```python
from build123d import *

# Parameters (mm, degrees)
F0_W     = 7
F0_H     = 5
F0_H_2   = 1
F0_W_2   = 10
F0_W_3   = 5
F0_H_3   = 2.5
F1_DEPTH = 30


with BuildPart() as f1:
    # F0 (on Top) → F1 (new body)
    with BuildSketch(Plane.XY):
        with BuildLine():
            Line((20, 12.5), (20, 17.5))
            Line((20, 17.5), (-13, 17.5))
            Line((-13, 17.5), (-13, 12.5))
            Line((-13, 12.5), (-8.2915619759, 12.5))
            ThreePointArc((-8.2915619759, 12.5), (0, 15), (8.2915619759, 12.5))
            Line((8.2915619759, 12.5), (20, 12.5))
        make_face()
        with Locations((23.5, 15)):
            Rectangle(F0_W, F0_H)
        with Locations((-16.5, 15)):
            Rectangle(F0_W, F0_H)
        with Locations((23.5, 12)):
            Rectangle(F0_W, F0_H_2)
        with BuildLine():
            Line((20, 11.5), (20, 12.5))
            Line((20, 12.5), (8.2915619759, 12.5))
            ThreePointArc((8.2915619759, 12.5), (13.2169101843, 7.0931858273), (15, 0))
            ThreePointArc((15, 0), (13.2169101843, -7.0931858273), (8.2915619759, -12.5))
            Line((8.2915619759, -12.5), (20, -12.5))
            Line((20, -12.5), (20, -11.5))
            Line((20, -11.5), (20, 11.5))
        make_face()
        with Locations((32, 15)):
            Rectangle(F0_W_2, F0_H)
        with BuildLine():
            Line((-13, 7.4833147735), (-13, 12.5))
            Line((-13, 12.5), (-20, 12.5))
            Line((-20, 12.5), (-20, 5))
            Line((-20, 5), (-14.1421356237, 5))
            ThreePointArc((-14.1421356237, 5), (-13.627750901, 6.2677272898), (-13, 7.4833147735))
        make_face()
        with BuildLine():
            Line((-8.2915619759, 12.5), (-13, 12.5))
            Line((-13, 12.5), (-13, 7.4833147735))
            ThreePointArc((-13, 7.4833147735), (-10.9372956213, 10.2652600791), (-8.2915619759, 12.5))
        make_face()
        with BuildLine():
            Line((-8.2915619759, 12.5), (8.2915619759, 12.5))
            ThreePointArc((8.2915619759, 12.5), (0, 15), (-8.2915619759, 12.5))
        make_face()
        with BuildLine():
            Line((-13, 5), (-13, 7.4833147735))
            ThreePointArc((-13, 7.4833147735), (-13.627750901, 6.2677272898), (-14.1421356237, 5))
            Line((-14.1421356237, 5), (-13, 5))
        make_face()
        with Locations((23.5, -12)):
            Rectangle(F0_W, F0_H_2)
        with Locations((23.5, -15)):
            Rectangle(F0_W, F0_H)
        with BuildLine():
            Line((20, -17.5), (20, -12.5))
            Line((20, -12.5), (8.2915619759, -12.5))
            ThreePointArc((8.2915619759, -12.5), (4.3301270189, -14.3614066163), (0, -15))
            Line((0, -15), (-15, -15))
            Line((-15, -15), (-15, -17.5))
            Line((-15, -17.5), (20, -17.5))
        make_face()
        with BuildLine():
            ThreePointArc((0, -15), (4.3301270189, -14.3614066163), (8.2915619759, -12.5))
            Line((8.2915619759, -12.5), (-8.2915619759, -12.5))
            ThreePointArc((-8.2915619759, -12.5), (-4.3301270189, -14.3614066163), (0, -15))
        make_face()
        with Locations((-17.5, -11.25)):
            Rectangle(F0_W_3, F0_H_3)
        with BuildLine():
            ThreePointArc((0, -15), (-4.3301270189, -14.3614066163), (-8.2915619759, -12.5))
            Line((-8.2915619759, -12.5), (-15, -12.5))
            Line((-15, -12.5), (-15, -15))
            Line((-15, -15), (0, -15))
        make_face()
        Polygon((-15, -12.5), (-20, -12.5), (-20, -17.5), (-15, -17.5), (-15, -15), align=None)
    extrude(amount=F1_DEPTH)


solid = f1.part
```
The listing builds one solid part. Answer for the finished solid, in the listing's coordinates (mm). A direction names the side the tool comes from. Coordinates: 2 decimals unless noted, no trailing zeros. Loops run counter-clockwise (first coordinate to the right, second up) from the corner with the lowest first, then second, coordinate; pieces in that order, holes last. Notation, with made-up numbers: (-8.5, 21.5) - (22.5, 21.5) arc R18 cw to (22.5, 50.5) - close; hole circle Ø11 at (85.25, 26). An arc over 180 degrees is marked (long way). Use a Markdown table: item, result. Add a question column.
1) The part is cut by section B-B, the plane z = 24.75. Give the vertices of the cut face in (x, y).
2) The mould has two halves that part along X. Classify faces 1 (the flat face through (27, -15, 15)), 2 (the flat face through (0, 12.5, 15)), 3 (the flat face through (23, 11.5, 15)), 4 (the flat face through (-3, -12.5, 15)): released by +X, released by -X, zero draft, split by the parting line, or undercut.
3) The part is cut by section D-D, the plane y = -14.5. Give the vertices of the cut face in (x, z), and give its area (3 significant figures).
4) The part is cut by section C-C, the plane x = 30.5. Give the vertices of the cut face in (y, z), and give its area (3 significant figures).
5) For faces 5 (the flat face through (-18, -10, 15)), 6 (the flat face through (-15, -11, 15)), 7 (the flat face through (20, 0, 15)), determine the directions among +Z, -Z, +X, -X, +Y, -Y from which every point of the face is accessible in a straight line to the end or side of a thin tool.
6) Given pin 1 (2 mm diameter, centred on x = 12, y = 12.5, fed in from -Z); pin 2 (3 mm diameter, centred on y = -10.5, z = 8.5, fed in from +X); pin 3 (3 mm diameter, centred on y = 0.5, z = 9.5, fed in from +X); pin 4 (1.5 mm diameter, centred on y = 1.5, z = 20, fed in from -X), each flat-ended and moving along its own axis, determine where each tip first touches the part or whether it passes through.
7) Find the intervals of material crossed by line 1 (Y direction, x = 25, z = 3.25); line 2 (Y direction, x = -0.5, z = 3.75); line 3 (Y direction, x = 34, z = 1.5), in increasing order.
8) The part is cut by section A-A, the plane x = 4.5. Give the vertices of the cut face in (y, z).
Here are the results:
| question | item | result |
|---|---|---|
| 1 | outline | (-20, -17.5) - (27, -17.5) - (27, -11.5) - (20, -11.5) - (20, 11.5) - (27, 11.5) - (27, 12.5) - (37, 12.5) - (37, 17.5) - (-20, 17.5) - (-20, 5) - (-13, 5) - (-13, 7.48) arc R15 cw to (-8.29, 12.5) - (8.29, 12.5) arc R15 cw to (8.29, -12.5) - (-15, -12.5) - (-15, -10) - (-20, -10) - close |
| 2 | face 1 | released by +X |
| 2 | face 2 | undercut |
| 2 | face 3 | zero draft |
| 2 | face 4 | undercut |
| 3 | outline | (-20, 0) - (27, 0) - (27, 30) - (-20, 30) - close |
| 3 | area | 1,410 mm^2 |
| 4 | outline | (12.5, 0) - (17.5, 0) - (17.5, 30) - (12.5, 30) - close |
| 4 | area | 150 mm^2 |
| 5 | face 5 | +Z, -Z, -X |
| 5 | face 6 | +Z, -Z |
| 5 | face 7 | +Z, -Z, +X |
| 6 | pin 1 | stops at z = 0 |
| 6 | pin 2 | stops at x = 27 |
| 6 | pin 3 | stops at x = 20 |
| 6 | pin 4 | stops at x = 14.83 |
| 7 | line 1 | y = -17.5 to -11.5, 11.5 to 17.5 |
| 7 | line 2 | y = -17.5 to -12.5, 12.5 to 17.5 |
| 7 | line 3 | y = 12.5 to 17.5 |
| 8 | outline | (-17.5, 0) - (-12.5, 0) - (-12.5, 30) - (-17.5, 30) - close; (12.5, 0) - (17.5, 0) - (17.5, 30) - (12.5, 30) - close |
